Part model, mm, in its own coordinate system. Face numbers are marked on the shaded views. A direction names the side the tool comes from. Round coordinates to 2 decimals unless told otherwise and drop trailing zeros. Write each loop counter-clockwise with the first axis right and the second up, starting at its lowest first coordinate (ties: lowest second). Pieces come first, ordered by that corner, then holes.
1) Saw through at C-C on z = 30.5. Write the cut outline in (x, y), and give its area (3 significant figures).
2) Which spindle directions (+Z, -Z, +X, -X, +Y, -Y) get a long thin tool onto all of the face, cutting with end or side? Do the marked faces 1, 2, 3, 4 and 5. Say none if no direction does.
3) Flat gauge pins, fed straight in: pin 1 (2.5 mm diameter, centred on x = 26.5, y = -4.5, fed in from +Z); pin 2 (4 mm diameter, centred on y = -3, z = 15, fed in from -X); pin 3 (6.5 mm diameter, centred on y = -0.5, z = 36, fed in from +X); pin 4 (1 mm diameter, centred on x = 7.5, y = 6.5, fed in from -Z). Where does each tip first touch, or does it go through?
4) Saw through at D-D on x = 21. Write the cut outline in (y, z).
5) Saw through at B-B on y = 0. Write the cut outline in (x, z).
6) Drill centre lines: L1, parallel to X at y = 1, z = 4; L2, parallel to Z at x = -14.5, y = -0.25; L3, parallel to Z at x = -23, y = 3. Where is each one in solid material? Low to high.
7) Saw through at A-A on y = 6. Write the cut outline in (x, z), and give its area (3 significant figures).
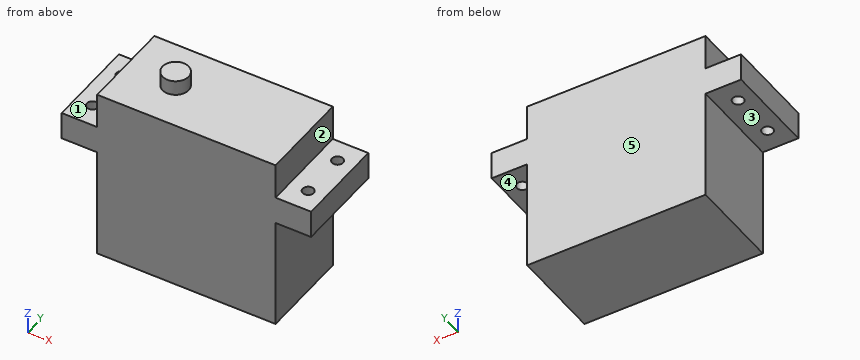
```python
from build123d import *

# Parameters (mm, degrees)
SKETCH1_W                    = 56.8198
SKETCH1_H                    = 20.9804
EXTRUDE1_DEPTH               = 43.2816
SKETCH3_OUTSIDE_W            = 73.708
SKETCH3_OUTSIDE_H            = 37.868
SKETCH3_OUTSIDE_R            = 2.9718
EXTRUDE2_DEPTH               = 3.4036
SKETCH8_W                    = 8.0899
SKETCH8_H                    = 20.9804
EXTRUDE5_DEPTH               = 25.4
F_39_0_0995_DIAMETER_HOLE1_D = 2.5273
SKETCH13_W                   = 8.0899
SKETCH13_H                   = 20.9804
EXTRUDE6_DEPTH               = 8.128


with BuildPart() as part:
    # Sketch1 → Extrude1 (new body)
    with BuildSketch(Plane.XY):
        Rectangle(SKETCH1_W, SKETCH1_H)
    extrude(amount=EXTRUDE1_DEPTH)

    # Sketch3 outside → Extrude2 (cut)
    with BuildSketch(Plane.XY.offset(43.2816)):
        Rectangle(SKETCH3_OUTSIDE_W, SKETCH3_OUTSIDE_H)
        with Locations((-8.9789, 0)):
            Circle(SKETCH3_OUTSIDE_R, mode=Mode.SUBTRACT)
    extrude(amount=-EXTRUDE2_DEPTH, mode=Mode.SUBTRACT)

    # Sketch8 → Extrude5 (cut)
    with BuildSketch(Plane(origin=(0, 0, 0), x_dir=(-1, 0, 0), z_dir=(0, 0, -1))):
        with Locations((-24.36495, 0)):
            Rectangle(SKETCH8_W, SKETCH8_H)
        with Locations((24.36495, 0)):
            Rectangle(SKETCH8_W, SKETCH8_H)
    extrude(amount=-EXTRUDE5_DEPTH, mode=Mode.SUBTRACT)

    # #39 (0.0995) Diameter Hole1 (through all)
    with Locations(Plane(origin=(-24.5745, 5.3975, 39.878), x_dir=(1, 0, 0), z_dir=(0, 0, 1))):
        with Locations((0, 0), (0, -10.795), (49.149, 0), (49.149, -10.795)):
            Hole(F_39_0_0995_DIAMETER_HOLE1_D / 2)

    # Sketch13 → Extrude6 (cut)
    with BuildSketch(Plane.XY.offset(39.878)):
        with Locations((-24.36495, 0)):
            Rectangle(SKETCH13_W, SKETCH13_H)
        with Locations((24.36495, 0)):
            Rectangle(SKETCH13_W, SKETCH13_H)
    extrude(amount=-EXTRUDE6_DEPTH, mode=Mode.SUBTRACT)


solid = part.part
```
Completed:
1. outline: (-28.41, -10.49) - (28.41, -10.49) - (28.41, 10.49) - (-28.41, 10.49) - close; hole circle Ø2.53 at (-24.57, -5.4); hole circle Ø2.53 at (-24.57, 5.4); hole circle Ø2.53 at (24.57, -5.4); hole circle Ø2.53 at (24.57, 5.4)
1. area: 1,170 mm2
2. face 1: +Z, -X, +Y, -Y
2. face 2: +Z, +X, +Y, -Y
2. face 3: -Z, -X, +Y, -Y
2. face 4: -Z, +X, +Y, -Y
2. face 5: +Z, -Z, +X, -X, +Y
3. pin 1: stops at z = 31.75
3. pin 2: stops at x = -20.32
3. pin 3: stops at x = 20.32
3. pin 4: stops at z = 0
4. outline: (-10.49, 25.4) - (10.49, 25.4) - (10.49, 31.75) - (-10.49, 31.75) - close
5. outline: (-28.41, 25.4) - (-20.32, 25.4) - (-20.32, 0) - (20.32, 0) - (20.32, 25.4) - (28.41, 25.4) - (28.41, 31.75) - (20.32, 31.75) - (20.32, 39.88) - (-6.01, 39.88) - (-6.01, 43.28) - (-11.95, 43.28) - (-11.95, 39.88) - (-20.32, 39.88) - (-20.32, 31.75) - (-28.41, 31.75) - close
6. L1: x = -20.32 to 20.32
6. L2: z = 0 to 39.88
6. L3: z = 25.4 to 31.75
7. outline: (-28.41, 25.4) - (-25.69, 25.4) - (-25.69, 31.75) - (-28.41, 31.75) - close; (-23.46, 25.4) - (-20.32, 25.4) - (-20.32, 0) - (20.32, 0) - (20.32, 25.4) - (23.46, 25.4) - (23.46, 31.75) - (20.32, 31.75) - (20.32, 39.88) - (-20.32, 39.88) - (-20.32, 31.75) - (-23.46, 31.75) - close; (25.69, 25.4) - (28.41, 25.4) - (28.41, 31.75) - (25.69, 31.75) - close
7. area: 1,700 mm2
